Autodesk Inventor part; units mm, degrees
ref_plane "YZ Plane" through (0, 0, 0) normal (1, 0, 0) x (0, 1, 0)
ref_plane "XZ Plane" through (0, 0, 0) normal (0, 1, 0) x (-1, 0, 0)
ref_plane "XY Plane" through (0, 0, 0) normal (0, 0, 1) x (1, 0, 0)
sketch "Sketch1" plane through (0, 0, 0) normal (0, 0, 1) x (1, 0, 0)
  line L0 (-11.6758, 23.572) -> (2.2942, 23.572)
  line L1 (2.2942, 23.572) -> (8.0092, 17.222)
  line L2 (8.0092, 17.222) -> (8.0092, -20.878)
  line L3 (8.0092, -20.878) -> (2.2942, -27.228)
  line L4 (2.2942, -27.228) -> (-11.6758, -27.228)
  line L5 (-11.6758, -27.228) -> (-17.3908, -20.878)
  line L6 (-17.3908, -20.878) -> (-17.3908, 17.222)
  line L7 (-17.3908, 17.222) -> (-11.6758, 23.572)
  line L8 (-4.6908, 23.572) -> (-4.6908, -27.228) construction
  line L9 (-17.3908, -1.828) -> (8.0092, -1.828) construction
  dimension "d0" = 25.4
  dimension "d1" = 50.8
  dimension "d2" = 5.715
  dimension "d4" = 6.35
extrude "Extrusion1" add sketch "Sketch1" along normal blind 3.175
sketch "Sketch2" plane through (0, 0, 3.175) normal (0, 0, 1) x (1, 0, 0)
  line L0 (-17.3908, -20.878) -> (-17.3908, 17.222)
  line L1 (8.0092, 17.222) -> (8.0092, -20.878)
  line L2 (-17.3908, 10.872) -> (8.0092, 10.872)
  line L3 (-17.3908, -14.528) -> (8.0092, -14.528)
  point P0 (2.2942, -27.228)
  dimension "d11" = 25.4
  dimension "d12" = 12.7
extrude "Extrusion2" add sketch "Sketch2" against normal blind 8.89
sketch "Sketch3" plane through (0, 0, -5.715) normal (0, 0, -1) x (-1, 0, 0)
  line L0 (17.3908, -14.528) -> (-8.0092, -14.528)
  line L1 (-8.0092, 10.872) -> (17.3908, 10.872)
  line L2 (-8.0092, -14.528) -> (-8.0092, 10.872)
  line L3 (-2.2942, 3.887) -> (11.6758, 3.887)
  line L4 (11.6758, 3.887) -> (11.6758, -7.543)
  line L5 (11.6758, -7.543) -> (-2.2942, -7.543)
  line L6 (-2.2942, -7.543) -> (-2.2942, 3.887)
  circle A0 centre (4.6908, -1.828) radius 5.715 construction
  circle A1 centre (4.6908, -1.828) radius 12.7 construction
  dimension "d15" = 11.43
  dimension "d16" = 5.715
  dimension "d17" = 5.715
extrude "Extrusion3" cut sketch "Sketch3" against normal through all
sketch "Sketch4" plane through (0, 0, -5.715) normal (0, 0, -1) x (-1, 0, 0)
  line L0 (11.6758, 3.887) -> (11.6758, -7.543)
  line L1 (-2.2942, 3.887) -> (11.6758, 3.887)
  line L2 (11.6758, 3.887) -> (11.6758, 5.157)
  line L3 (11.6758, 5.157) -> (-2.2942, 5.157)
  line L4 (-2.2942, 5.157) -> (-2.2942, 3.887)
  line L5 (-2.2942, -7.543) -> (11.6758, -7.543)
  line L6 (11.6758, -7.543) -> (11.6758, -8.813)
  line L7 (11.6758, -8.813) -> (-2.2942, -8.813)
  line L8 (-2.2942, -8.813) -> (-2.2942, -7.543)
  dimension "d20" = 1.27
  dimension "d21" = 1.27
extrude "Extrusion4" add sketch "Sketch4" along normal blind 3.81
sketch "Sketch5" plane through (0, 0, 3.175) normal (0, 0, 1) x (1, 0, 0)
  line L0 (2.2942, 3.887) -> (2.2942, -7.543)
  line L1 (2.2942, -7.543) -> (-11.6758, -7.543)
  line L2 (-11.6758, -7.543) -> (-11.6758, 3.887)
  line L3 (-11.6758, 3.887) -> (2.2942, 3.887)
  line L4 (-14.2158, 7.697) -> (4.8342, 7.697)
  line L5 (4.8342, 7.697) -> (4.8342, -11.353)
  line L6 (4.8342, -11.353) -> (-14.2158, -11.353)
  line L7 (-14.2158, -11.353) -> (-14.2158, 7.697)
  point P0 (-17.3908, -20.878)
  point P1 (-11.6758, 23.572)
  dimension "d24" = 19.05
  dimension "d25" = 19.05
  dimension "d26" = 3.175
  dimension "d27" = 15.875
extrude "Extrusion5" cut sketch "Sketch5" against normal blind 6.35
sketch "Sketch6" plane through (-17.3908, -20.878, 3.175) normal (-1, 0, 0) x (0, 0, 1)
  line L0 (-4.699, 26.67) -> (-3.175, 26.67)
  line L1 (-3.175, 26.67) -> (-3.175, 11.43)
  line L2 (-3.175, 11.43) -> (-4.699, 11.43)
  line L3 (-4.699, 11.43) -> (-4.699, 26.67)
  line L4 (-3.175, 44.45) -> (0, 44.45)
  point P0 (0, 0)
  dimension "d30" = 15.24
  dimension "d31" = 1.524
  dimension "d32" = 3.175
  dimension "d33" = 17.78
extrude "Extrusion6" cut sketch "Sketch6" against normal through all
fillet "Fillet1" radius 2.54 4 edges at (2.2942, -8.178, -9.525) (2.2942, 4.522, -9.525) (-11.6758, 4.522, -9.525) (-11.6758, -8.178, -9.525)
sketch "Sketch7" plane through (-11.6758, -8.813, -5.715) normal (0, -1, 0) x (1, 0, 0)
  line L0 (-5.715, 5.715) -> (-5.715, 0)
  line L1 (0, 8.89) -> (-5.715, 8.89)
  point P0 (7.62, -1.905)
  dimension "d37" = 13.335
  dimension "d38" = 10.795
hole "Hole1" at (-4.0558, -8.813, -7.62) direction (0, 1, 0) diameter 2.54 end through all
sketch "Sketch8" plane through (0, 0, 0) normal (0, 0, -1) x (-1, 0, 0)
  line L0 (-8.0092, 17.222) -> (-8.0092, 10.872)
  line L1 (11.6758, 23.572) -> (-2.2942, 23.572)
  point P0 (4.6908, 17.222)
  point P1 (4.6908, -20.878)
  dimension "d46" = 12.7
  dimension "d47" = 6.35
  dimension "d48" = 38.1
hole "Hole2" at (-4.6908, 17.222, 0) at (-4.6908, -20.878, 0) direction (0, 0, 1) diameter 4.064 end through all countersink diameter 6.35 countersink angle 82
properties part number "latchbase"
Design review of the part built by this model. Coordinates are the model's own, in mm. A direction names the side the tool comes from. Round coordinates to 2 decimals unless told otherwise and drop trailing zeros. Order: outer loops, then holes, each group sorted by start corner. A loop starts at its lowest first (then second) coordinate and runs counter-clockwise, first axis right, second up. Notation, with made-up numbers: (-22.5, 89) - (6.5, 89) arc R10 ccw to (6.5, 94) - close; hole circle Ø6 at (-29, 39). An arc over 180 degrees is marked (long way). Return JSON: item names as keys, results as strings.
Q1. The part is to be moulded in two halves that separate along Z. For faces 5 (the flat face through (2.294, 5, -6)), 6 (the flat face through (6, -9.448, -1)), 7 (the cylindrical face through (-10.91, 4.53, -8.8)), say which applies: pulls with the +Z half, pulls with the -Z half, needs draft (parallel to the pull), parting line crosses it, or undercut.
Computed values:
{"face 5": "needs draft", "face 6": "undercut", "face 7": "pulls with the -Z half"}
Q2. Consider section C-C on x = -10. Write out the cut boundary in (y, z) (3 decimals).
Computed values:
{"outline": "(-27.228, 0) - (-14.528, 0) - (-14.528, -5.715) - (-8.813, -5.715) - (-8.813, -9.373) - (-7.543, -9.373) - (-7.543, -3.175) - (-11.353, -3.175) - (-11.353, 3.175) - (-27.228, 3.175) - close; (3.887, -9.373) - (5.157, -9.373) - (5.157, -5.715) - (10.872, -5.715) - (10.872, 0) - (23.572, 0) - (23.572, 3.175) - (7.697, 3.175) - (7.697, -3.175) - (3.887, -3.175) - close"}
Q3. Wall thickness on L1, parallel to X at y = -1.5, z = 0.25; L2, parallel to X at y = -7.5, z = -3.25; L3, parallel to Y at x = -1.5, z = -3: over which ranges is each line inside the solid? List them lowest first. Write a range as [from, to].
Computed values:
{"L1": "x = [-17.39, -14.22], [4.83, 8.01]", "L2": "x = [-17.39, -11.68], [2.29, 8.01]", "L3": "y = [-14.53, -11.35], [7.7, 10.87]"}
Q4. Consider section A-A on y = -2. Write out the cut boundary in (x, z) (3 decimals).
Computed values:
{"outline": "(-17.391, -5.715) - (-11.676, -5.715) - (-11.676, -3.175) - (-14.216, -3.175) - (-14.216, -1.524) - (-17.391, -1.524) - close; (-17.391, 0) - (-14.216, 0) - (-14.216, 3.175) - (-17.391, 3.175) - close; (2.294, -5.715) - (8.009, -5.715) - (8.009, -1.524) - (4.834, -1.524) - (4.834, -3.175) - (2.294, -3.175) - close; (4.834, 0) - (8.009, 0) - (8.009, 3.175) - (4.834, 3.175) - close"}
Q5. For pin 1 Ø4.5 at (x, z) = (-6, -3.5) entering from +Y; pin 2 Ø5 at (x, z) = (-4, -7.5) entering from -Y; pin 3 Ø2 at (x, z) = (-13.5, 1.5) entering from -Y, all flat-tipped, find the tip position at first contact; note any pin that passes through.
Computed values:
{"pin 1": "stops at y = 10.87", "pin 2": "stops at y = -14.53", "pin 3": "stops at y = -26.31"}
Q6. Consider section D-D on z = -4.5. Write out the cut boundary in (x, y), plus the area to 3 significant figures.
Computed values:
{"outline": "(-17.39, -14.53) - (8.01, -14.53) - (8.01, 10.87) - (-17.39, 10.87) - close; hole (-11.68, -7.54) - (2.29, -7.54) - (2.29, 3.89) - (-11.68, 3.89) - close", "area": "485 mm2"}
Q7. Consider section B-B on z = -8.25. Write out the cut boundary in (x, y), plus the area to 3 significant figures.
Computed values:
{"outline": "(-11.34, -8.81) - (-5.16, -8.81) - (-5.16, -7.54) - (-11.34, -7.54) - close; (-11.34, 3.89) - (-5.16, 3.89) - (-5.16, 5.16) - (-11.34, 5.16) - close; (-2.95, -8.81) - (1.96, -8.81) - (1.96, -7.54) - (-2.95, -7.54) - close; (-2.95, 3.89) - (1.96, 3.89) - (1.96, 5.16) - (-2.95, 5.16) - close", "area": "28.2 mm2"}
Q8. Machinability: for faces 1 (the flat face through (-5, -14.528, -3)), 2 (the flat face through (-5, 10.872, -3)), 3 (the flat face through (-5, 5, -3.175)), 4 (the flat face through (-11.676, -8, -6)), which of the approach directions +Z, -Z, +X, -X, +Y, -Y give a long, thin tool a straight path to every point of the face, cutting with its end or side? Answer none if there is none.
Computed values:
{"face 1": "-Z, +X, -X, -Y", "face 2": "-Z, +X, -X, +Y", "face 3": "+Z", "face 4": "-Z, -X, +Y, -Y"}
